Check sheet for the modelled part. Datum: model origin and axes. Units: mm. A direction names the side the tool comes from. Coordinates: 2 decimals unless noted, no trailing zeros. Loops run counter-clockwise (first coordinate to the right, second up) from the corner with the lowest first, then second, coordinate; pieces in that order, holes last. Notation, with made-up numbers: (60.25, 85.5) -> (87.25, 85.5) arc R12 cw to (87.25, 90.5) -> close; hole circle Ø3 at (42.25, -27.75). An arc over 180 degrees is marked (long way). Use CSV: the item, a comma, the result in double quotes. Start each with the question number.
1. Sectioned sample at B-B, the plane x = -39. Record the cut outline in (y, z).
2. Sectioned sample at C-C, the plane y = 82.5. Record the cut outline in (x, z).
3. Sectioned sample at A-A, the plane z = 6.5. Record the cut outline in (x, y).
4. Thickness scan on L1, parallel to Y at x = 29, z = 5.75; L2, parallel to X at y = 102, z = 10.5; L3, parallel to X at y = 111.5, z = 5.25. Record the ranges inside material, lowest first.
5. Gauge pin test, flat end, axial feed: pin 1 (2 mm diameter, centred on x = -33.5, y = 91, fed in from +Z). Record the tip position at first contact, or that the pin passes through.
6. Release check for a two-part mould opening along Y. For faces 3 (the face through (-61.301, 36, 6)), 4 (the face through (37.49, -37.71, 6.41)), 5 (the face through (-9, -44.126, 6)), 6 (the face through (-59.798, 116.206, 6.591)) record: pulls with the +Y half, pulls with the -Y half, needs draft (parallel to the pull), parting line crosses it, or undercut.
7. Set-up check for faces 1 (the face through (32.801, 38, 8)), 2 (the face through (-10, 117.632, 6)): record each of +Z, -Z, +X, -X, +Y, -Y from which the full face is reachable in a straight line by a thin tool's end or side.
Autodesk Fusion 360 part; units mm, degrees
sketch "Sketch1" plane through (0, 0, 0) normal (0, 0, 1) x (1, 0, 0)
  line L0 (-51.3011, 107.6317) -> (32.8009, 107.6317)
  line L1 (32.8009, 107.6317) -> (32.8009, -34.1263)
  line L2 (32.8009, -34.1263) -> (-51.3011, -34.1263)
  line L3 (-51.3011, -34.1263) -> (-51.3011, 107.6317)
  line L4 (-61.3011, 117.6317) -> (42.8009, 117.6317)
  line L5 (42.8009, 117.6317) -> (42.8009, -44.1263)
  line L6 (42.8009, -44.1263) -> (-61.3011, -44.1263)
  line L7 (-61.3011, -44.1263) -> (-61.3011, 117.6317)
  circle A0 centre (37.8009, 112.6317) radius 1.45
  circle A1 centre (37.8009, -39.1263) radius 1.45
  circle A2 centre (-56.3011, -39.1263) radius 1.45
  circle A3 centre (-56.3011, 112.6317) radius 1.45
  dimension "d1" = 84.102
  dimension "d2" = 141.758
  dimension "d3" = 104.102
  dimension "d4" = 161.758
  dimension "d5" = 10
  dimension "d6" = 10
  dimension "d7" = 2.9
  dimension "d8" = 5
  dimension "d9" = 5
  dimension "d10" = 2.9
  dimension "d11" = 5
  dimension "d12" = 5
  dimension "d13" = 2.9
  dimension "d14" = 5
  dimension "d15" = 5
  dimension "d16" = 2.9
  dimension "d17" = 5
  dimension "d18" = 5
extrude "Extrude1" add sketch "Sketch1" along normal blind 3 contours L0 L1 L2 L3
extrude "Extrude2" add sketch "Sketch1" along normal blind 13
fillet "Fillet1" radius 5 4 edges at (42.8009, -44.1263, 6.5) (42.8009, 117.6317, 6.5) (-61.3011, 117.6317, 6.5) (-61.3011, -44.1263, 6.5)
Completed:
1,outline,"(-44.13, 0) -> (117.63, 0) -> (117.63, 13) -> (107.63, 13) -> (107.63, 3) -> (-34.13, 3) -> (-34.13, 13) -> (-44.13, 13) -> close"
2,outline,"(-61.3, 0) -> (42.8, 0) -> (42.8, 13) -> (32.8, 13) -> (32.8, 3) -> (-51.3, 3) -> (-51.3, 13) -> (-61.3, 13) -> close"
3,outline,"(-61.3, -39.13) arc R5 ccw to (-56.3, -44.13) -> (37.8, -44.13) arc R5 ccw to (42.8, -39.13) -> (42.8, 112.63) arc R5 ccw to (37.8, 117.63) -> (-56.3, 117.63) arc R5 ccw to (-61.3, 112.63) -> close; hole circle Ø2.9 at (-56.3, -39.13); hole circle Ø2.9 at (-56.3, 112.63); hole (-51.3, -34.13) -> (32.8, -34.13) -> (32.8, 107.63) -> (-51.3, 107.63) -> close; hole circle Ø2.9 at (37.8, -39.13); hole circle Ø2.9 at (37.8, 112.63)"
4,L1,"-44.13 to -34.13, 107.63 to 117.63"
4,L2,"-61.3 to -51.3, 32.8 to 42.8"
4,L3,"-61.3 to -57.21, -55.39 to 36.89, 38.71 to 42.8"
5,pin 1,"z = 3"
6,face 3,"needs draft"
6,face 4,"undercut"
6,face 5,"pulls with the -Y half"
6,face 6,"pulls with the +Y half"
7,face 1,"+Z"
7,face 2,"+Z, -Z, +X, -X, +Y"
